For this review, take the finished solid that the model builds, in its own axes (mm). Face numbers are marked on the shaded views. A direction names the side the tool comes from. Coordinates: 2 decimals unless noted, no trailing zeros. Write each loop counter-clockwise with the first axis right and the second up, starting at its lowest first coordinate (ties: lowest second). Pieces come first, ordered by that corner, then holes.
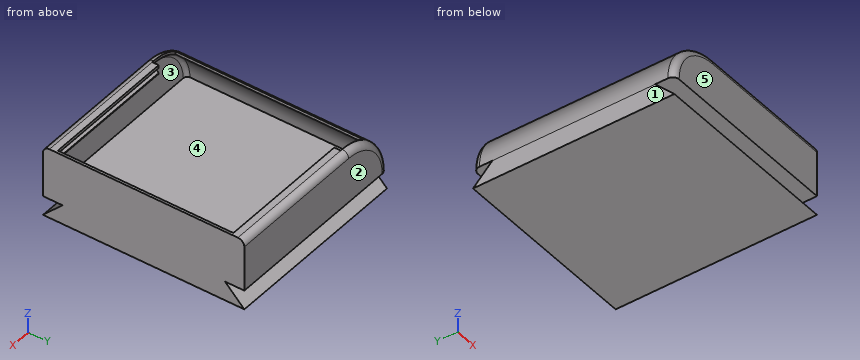
```python
from build123d import *

# Parameters (mm, degrees)
SKETCH1_W            = 148.500856602
SKETCH1_H            = 156
BOSS_EXTRUDE1_DEPTH  = 40
FILLET3_R            = 40
FILLET4_R            = 5
SHELL4_T             = -2
SKETCH19_W           = 131
SKETCH19_H           = 146
CUT_EXTRUDE8_DEPTH   = 10
SKETCH21_W           = 107
SKETCH21_H           = 2
BOSS_EXTRUDE7_DEPTH  = 5
BOSS_EXTRUDE8_START  = -107
BOSS_EXTRUDE8_DEPTH  = 107
CUT_EXTRUDE9_DEPTH   = 107
BOSS_EXTRUDE9_DEPTH  = 2
BOSS_EXTRUDE10_DEPTH = 15
CUT_EXTRUDE10_DEPTH  = 170
SHELL5_START         = -57.680419874
SHELL5_DEPTH         = 103
SKETCH29_W           = 7.658063704
SKETCH29_H           = 119.773909492
CUT_EXTRUDE11_DEPTH  = 170
SKETCH31_W           = 7.658063704
SKETCH31_H           = 119.773909492
BOSS_EXTRUDE12_DEPTH = 2
SKETCH32_W           = 7.658063704
SKETCH32_H           = 119.773909492
BOSS_EXTRUDE13_DEPTH = 2


# Read off the part's stored shape, not the designer's step: Shell5
# Some blends are built 0.0001 mm under size
with BuildPart() as part:
    # Sketch1 → Boss-Extrude1 (new body)
    with BuildSketch(Plane.XY):
        with Locations((-26.930848175, -80)):
            Rectangle(SKETCH1_W, SKETCH1_H)
    extrude(amount=BOSS_EXTRUDE1_DEPTH)

    # Fillet3
    fillet3_edges = [part.edges().sort_by_distance(p)[0] for p in [
        (-101.181276476, -80, 40),
    ]]
    fillet(fillet3_edges, radius=FILLET3_R - 0.0001)  # a hair under: the kernel refuses the full size

    # Fillet4
    # the kernel refuses this fillet: 5 mm, written as the material it takes off along each edge
    with BuildSketch(Plane(origin=(-61.181376476, -158, 40), x_dir=(0, 1, 0), z_dir=(1, 0, 0))) as fillet4_piece_1:
        with BuildLine():
            CenterArc((FILLET4_R, -FILLET4_R), FILLET4_R, 90, 90)
            Line((0, -FILLET4_R), (0, 0))
            Line((0, 0), (FILLET4_R, 0))
        make_face()
    extrude(amount=121.000956602, mode=Mode.SUBTRACT)
    with BuildSketch(Plane(origin=(-61.181376476, -158, 0.0001), x_dir=(-1, 0, 0), z_dir=(0, 0, -1))) as fillet4_piece_2:
        with BuildLine():
            CenterArc((39.9999 - FILLET4_R, FILLET4_R), FILLET4_R, 270, 90)
            Line((39.9999 - FILLET4_R, 0), (39.9999, 0))
            Line((39.9999, 0), (39.9999, FILLET4_R))
        make_face()
    revolve(axis=Axis((-61.181376476, -158, 0.0001), (0, 1, 0)), revolution_arc=90, mode=Mode.SUBTRACT)
    with BuildSketch(Plane(origin=(-61.181376476, -2, 0.0001), x_dir=(-1, 0, 0), z_dir=(0, 0, -1))) as fillet4_piece_3:
        with BuildLine():
            CenterArc((39.9999 - FILLET4_R, -FILLET4_R), FILLET4_R, 0, 90)
            Line((39.9999, -FILLET4_R), (39.9999, 0))
            Line((39.9999, 0), (39.9999 - FILLET4_R, 0))
        make_face()
    revolve(axis=Axis((-61.181376476, -2, 0.0001), (0, 1, 0)), revolution_arc=90, mode=Mode.SUBTRACT)
    with BuildSketch(Plane(origin=(59.819580126, -2, 40), x_dir=(0, 0, -1), z_dir=(-1, 0, 0))) as fillet4_piece_4:
        with BuildLine():
            CenterArc((FILLET4_R, FILLET4_R), FILLET4_R, 180, 90)
            Line((0, FILLET4_R), (0, 0))
            Line((0, 0), (FILLET4_R, 0))
        make_face()
    extrude(amount=121.000956602, mode=Mode.SUBTRACT)
    with BuildSketch(Plane(origin=(-101.181276476, -2, -12.5), x_dir=(1, 0, 0), z_dir=(0, 0, 1)), Plane(origin=(-101.181276476, -158, -12.5), x_dir=(0, 1, 0), z_dir=(0, 0, 1))) as fillet4_piece_5:
        with BuildLine():
            CenterArc((FILLET4_R, -FILLET4_R), FILLET4_R, 90, 90)
            Line((0, -FILLET4_R), (0, 0))
            Line((0, 0), (FILLET4_R, 0))
        make_face()
    extrude(amount=12.5001, mode=Mode.SUBTRACT)

    # Shell4
    shell4_openings = [part.faces().sort_by_distance(p)[0] for p in [
        (47.319580126, -80, 19.967473228),
    ]]
    offset(amount=SHELL4_T, openings=shell4_openings)

    # Sketch19 → Cut-Extrude8 (cut)
    with BuildSketch(Plane.XY.offset(40)):
        with Locations((-18.180419874, -80)):
            Rectangle(SKETCH19_W, SKETCH19_H)
    extrude(amount=-CUT_EXTRUDE8_DEPTH, mode=Mode.SUBTRACT)

    # Sketch21 → Boss-Extrude7 (add)
    with BuildSketch(Plane(origin=(0, -153, 0), x_dir=(1, 0, 0), z_dir=(0, 1, 0))):
        with Locations((-6.180419874, -39)):
            Rectangle(SKETCH21_W, SKETCH21_H)
    boss_extrude7 = extrude(amount=BOSS_EXTRUDE7_DEPTH)

    # Sketch22 → Boss-Extrude8 (add)
    with BuildSketch(Plane(origin=(47.319580126, 0, 0), x_dir=(0, 0, -1), z_dir=(1, 0, 0)).offset(BOSS_EXTRUDE8_START)):
        with BuildLine():
            Line((-38, -148), (-33, -148))
            Line((-33, -148), (-33, -156))
            Line((-33, -156), (-35, -156))
            ThreePointArc((-35, -156), (-37.121320344, -155.121320344), (-38, -153))
            Line((-38, -153), (-38, -148))
        make_face()
    boss_extrude8 = extrude(amount=BOSS_EXTRUDE8_DEPTH)

    # Sketch23 → Cut-Extrude9 (cut)
    with BuildSketch(Plane(origin=(47.319580126, 0, 0), x_dir=(0, 0, -1), z_dir=(1, 0, 0))):
        Polygon((-37.667948512, -148), (-37.667948512, -152.05), (-33.667948512, -148), align=None)
    cut_extrude9 = extrude(amount=-CUT_EXTRUDE9_DEPTH, mode=Mode.SUBTRACT)

    # Mirror1: Boss-Extrude7, Boss-Extrude8, Cut-Extrude9 across plane
    add(boss_extrude7.mirror(Plane.ZX.offset(-80)))
    add(boss_extrude8.mirror(Plane.ZX.offset(-80)))
    add(cut_extrude9.mirror(Plane.ZX.offset(-80)), mode=Mode.SUBTRACT)

    # Sketch25 → Boss-Extrude9 (add)
    with BuildSketch(Plane(origin=(47.319580126, 0, 0), x_dir=(0, 0, -1), z_dir=(1, 0, 0))):
        Polygon((-40, -148), (-37.667948512, -148), (-37.667948512, -152.05), (-33.667948512, -148), (-33, -148), (-33, -156), (-2, -156), (-2, -4), (-33, -4), (-33, -12), (-33.667948512, -12), (-37.667948512, -7.95), (-37.667948512, -12), (-40, -12), align=None)
    extrude(amount=-BOSS_EXTRUDE9_DEPTH)

    # Sketch26 → Boss-Extrude10 (add)
    with BuildSketch(Plane(origin=(0, 0, 0), x_dir=(-1, 0, 0), z_dir=(0, 0, -1))):
        Polygon((101.181276476, -7), (101.181276476, -153), (101.181276476, -158), (96.181276476, -158), (-47.319580126, -158), (-47.319580126, -2), (96.181276476, -2), (101.181276476, -2), align=None)
    extrude(amount=BOSS_EXTRUDE10_DEPTH)

    # Sketch27 → Cut-Extrude10 (cut)
    with BuildSketch(Plane.ZY.offset(101.181276476)):
        Polygon((0, -2), (0, -17), (-15, -2), align=None)
        Polygon((0, -158), (0, -143), (-15, -158), align=None)
    extrude(amount=-CUT_EXTRUDE10_DEPTH, mode=Mode.SUBTRACT)

    # Shell5 outline → Shell5 (cut)
    with BuildSketch(Plane.YZ.offset(SHELL5_START)):
        with BuildLine():
            Line((-152.194861825, 35), (-154.69858558, 37.472813585))
            ThreePointArc((-154.69858558, 37.472813585), (-155.654784053, 36.397183463), (-156, 35))
            Line((-156, 35), (-152.194861825, 35))
        make_face()
    extrude(amount=SHELL5_DEPTH, mode=Mode.SUBTRACT)

    # Sketch29 → Cut-Extrude11 (cut)
    with BuildSketch(Plane.ZY.offset(101.181276476)):
        with Locations((-8.13310084, -80.031899357)):
            Rectangle(SKETCH29_W, SKETCH29_H)
    extrude(amount=-CUT_EXTRUDE11_DEPTH, mode=Mode.SUBTRACT)

    # Sketch31 → Boss-Extrude12 (add)
    with BuildSketch(Plane(origin=(47.319580126, 0, 0), x_dir=(0, 0, -1), z_dir=(1, 0, 0))):
        with Locations((8.13310084, -80.031899357)):
            Rectangle(SKETCH31_W, SKETCH31_H)
    extrude(amount=-BOSS_EXTRUDE12_DEPTH)

    # Sketch32 → Boss-Extrude13 (add)
    with BuildSketch(Plane.ZY.offset(101.181276476)):
        with Locations((-8.13310084, -80.031899357)):
            Rectangle(SKETCH32_W, SKETCH32_H)
    extrude(amount=-BOSS_EXTRUDE13_DEPTH)


solid = part.part
```
Q1. Add section A-A (y = -120.5). State the section outline as (x, z) points.
Ans:
outline: (-101.18, -15) - (47.32, -15) - (47.32, 40) - (45.32, 40) - (45.32, 2) - (-99.13, 2) arc R38 cw to (-83.68, 30.62) - (-83.68, 33.07) arc R40 ccw to (-101.18, 0) - close; hole (-99.18, -11.96) - (45.32, -11.96) - (45.32, -4.3) - (-99.18, -4.3) - close
Q2. Draft analysis for pull direction Y (two halves, no side actions). For the marked faces 1, 2 and 3, state which applies: +Y half, -Y half, draft (parallel to the pull), parting line (faces both ways), or undercut.
Ans:
face 1: draft
face 2: +Y half
face 3: undercut
Q3. For probe 1 along Z at (x, y) = (13, -139); probe 2 along Y at (x, z) = (-8, 15.5); probe 3 along X at (y, z) = (-37, -11.5), list the stretches that pass through material, from the lowest coordinate up.
Ans:
probe 1: z = -15 to -11.96, -4.3 to 2
probe 2: y = -158 to -156, -4 to -2
probe 3: x = -101.18 to -99.18, 45.32 to 47.32
Q4. Tool access review of the marked faces 4 and 5: name each direction out of +Z, -Z, +X, -X, +Y, -Y from which nothing blocks a thin tool from reaching the whole face with its end or side.
Ans:
face 4: none
face 5: +Z, -Z, +X, -X, -Y
Q5. Add section B-B (z = -10). State the section outline as (x, y) points, then the cut area to 3 significant figures.
Ans:
outline: (-101.18, -153) - (47.32, -153) - (47.32, -7) - (-101.18, -7) - close; hole (-99.18, -139.92) - (45.32, -139.92) - (45.32, -20.14) - (-99.18, -20.14) - close
area: 4,370 mm2
Q6. Add section C-C (x = -22.5). Give the number of separate pieces and of enclosed holes in the cut face, then the cut area to 3 significant figures.
Ans:
separate pieces: 1
enclosed holes: 2
area: 1,740 mm2
Q7. Clearance check with flat-ended pins moving along their axes: pin 1 Ø8.5 at (x, z) = (-31.5, -9.5) entering from -Y; pin 2 Ø5 at (x, y) = (5, -78) entering from +Z; pin 3 Ø2 at (y, z) = (-10, 36) entering from -X. State where each tip first meets the part, or that it passes through.
Ans:
pin 1: stops at y = -156.75
pin 2: stops at z = 2
pin 3: stops at x = -59.68
